from build123d import *

# Parameters (mm, degrees)
F0_W     = 31.75
F0_H     = 6.35
F1_DEPTH = 12.7
F2_DEPTH = 3.175
F0_W_2   = 12.7


with BuildPart() as f1:
    # F0 (on Front) → F1 (new body, symmetric)
    with BuildSketch(Plane.XZ):
        Rectangle(F0_W, F0_H)
    extrude(amount=F1_DEPTH, both=True)

    # F0 (on Front) → F2 (join, symmetric)
    with BuildSketch(Plane.XZ):
        with BuildLine():
            Line((-15.875, 3.175), (15.875, 3.175))
            Line((15.875, 3.175), (15.875, 9.525))
            add(Edge.make_bspline(
                [(-15.875, 3.175), (-5.0392741859, 8.9093035005), (5.4355907996, 9.525), (15.875, 9.525)],
                knots=[0, 0, 0, 0, 32.3787739113, 32.3787739113, 32.3787739113, 32.3787739113], degree=3))
        make_face()
    extrude(amount=F2_DEPTH, both=True)

    # F0 (on Front) → F3 (revolve)
    with BuildSketch(Plane.XZ):
        with Locations((22.225, 6.35)):
            Rectangle(F0_W_2, F0_H)
    revolve(axis=Axis((15.875, 0, 6.35), (0, 0, 1)))


solid = f1.part
Input: part model. Units: mm. Frame: model coordinates. A direction names the side the tool comes from. Give positions to 0.01 mm unless a question says otherwise; leave off trailing zeros. Write each loop counter-clockwise with the first axis right and the second up, starting at its lowest first coordinate (ties: lowest second). Pieces come first, ordered by that corner, then holes. Notation, with made-up numbers: (28.5, -13) -> (82.5, -13) arc R8 cw to (82.5, -1) -> close; hole circle Ø9 at (-16, 24). An arc over 180 degrees is marked (long way). Use one line per item in the form item = value. Start each with the question number.
1) Pin query (flat end, axial travel): pin 1 (6 mm diameter, centred on x = 3, z = 7, fed in from -Y); pin 2 (5 mm diameter, centred on y = -5, z = 1.5, fed in from +X); pin 3 (1 mm diameter, centred on y = -5, z = 1.5, fed in from +X) (3 decimals). Return the tip coordinate at first contact, or that it passes through.
2) Ray query, probe 1 along X at (y, z) = (2, 2.75) (3 decimals); probe 2 along Z at (x, y) = (-1, 11) (3 decimals); probe 3 along Z at (x, y) = (22.5, 8.5) (3 decimals). Return the intervals inside material, ascending. Write a range as from..to.
3) Section query B-B on z = -0.75. Return the cut outline in (x, y) (3 decimals), then the cut area to 3 significant figures.
4) Section query C-C on x = 17. Return the cut outline in (y, z) (3 decimals).
5) Section query D-D on y = 6.25. Return the cut outline in (x, z) (3 decimals), then the cut area to 3 significant figures.
6) Set-up query: faces 1 (the flat face through (16, 0, 9.525)), 2 (the flat face through (15.875, 0, 0)), 3 (the flat face through (-4, 8, 3.175)), 4 (the flat face through (-4, -3.175, 5)), 5 (the cylindrical face through (27.99, 3.81, 6.39)). Return all of +Z, -Z, +X, -X, +Y, -Y with unobstructed straight access to the full face (end or side cutting, diameter ignored); none if empty.
7) Section query A-A on y = -4. Return the cut outline in (x, z) (3 decimals).
Outcome:
q1.pin_1 = -7.99
q1.pin_2 = 28.18
q1.pin_3 = 15.875
q2.probe_1 = -15.875..15.875
q2.probe_2 = -3.175..3.175
q2.probe_3 = 3.175..9.525
q3.outline = (-15.875, -12.7) -> (15.875, -12.7) -> (15.875, 12.7) -> (-15.875, 12.7) -> close
q3.area = 806 mm^2
q4.outline = (-12.65, 3.175) -> (12.65, 3.175) -> (12.65, 9.525) -> (-12.65, 9.525) -> close
q5.outline = (-15.875, -3.175) -> (15.875, -3.175) -> (15.875, 3.175) -> (26.931, 3.175) -> (26.931, 9.525) -> (4.819, 9.525) -> (4.819, 3.175) -> (-15.875, 3.175) -> close
q5.area = 342 mm^2
q6.face_1 = +Z, +X, -X, +Y, -Y
q6.face_2 = -Z, +X, +Y, -Y
q6.face_3 = +Z, -X, +Y
q6.face_4 = +Z, -X, -Y
q6.face_5 = +Z
q7.outline = (-15.875, -3.175) -> (15.875, -3.175) -> (15.875, 3.175) -> (27.929, 3.175) -> (27.929, 9.525) -> (3.821, 9.525) -> (3.821, 3.175) -> (-15.875, 3.175) -> close
